The model under review builds one solid part; all positions refer to its coordinate system, in mm. A direction names the side the tool comes from. Give positions to 0.01 mm unless a question says otherwise; leave off trailing zeros. Order: outer loops, then holes, each group sorted by start corner. A loop starts at its lowest first (then second) coordinate and runs counter-clockwise, first axis right, second up. Notation, with made-up numbers: (79, 4) - (125, 4) arc R7 cw to (125, 16) - close; hole circle Ø8 at (45.25, -26). An arc over 180 degrees is marked (long way). Write item = value, one per line. Start each with the question number.
1. Machinability: for faces 1 (the cylindrical face through (8.8, -3.65, 3.67)), 2 (the flat face through (-3.8, -4.4, 0)), which of the approach directions +Z, -Z, +X, -X, +Y, -Y give a long, thin tool a straight path to every point of the face, cutting with its end or side? Answer none if there is none.
2. We need section B-B, the plane x = 0. Give the boundary of the cut face in (y, z) (3 decimals), and give its area (3 significant figures).
3. We need section C-C, the plane z = 2.7. State how many separate pieces and enclosed holes the cut face has, and give its area (3 significant figures).
4. Mouldability with a two-part tool opening along X and no side actions: class faces 3 (the flat face through (10.582, -4.532, 1.565)), 4 (the flat face through (11, 1, 3.175)), 5 (the flat face through (-15.875, 0, 2)), 6 (the cylindrical face through (-14.05, -0.06, 1.57)) as pulls with the +X half, pulls with the -X half, needs draft (parallel to the pull), parting line crosses it, or undercut.
5. For P1, Ø1.5, axis at x = 11, y = 3, coming from the +Z side (3 decimals); P2, Ø9, axis at x = 0, y = 0, coming from the -Z side, all flat-tipped, find the tip position at first contact; note any pin that passes through.
6. We need section D-D, the plane y = -4.75. Give the boundary of the cut face in (x, z) (3 decimals), and give its area (3 significant figures).
7. We need section A-A, the plane y = 0. Give the boundary of the cut face in (x, z) (3 decimals), and give its area (3 significant figures).
8. Wall thickness on probe 1 along Y at (x, z) = (12.7, 1.1) (3 decimals); probe 2 along Y at (x, z) = (0, 1.75) (3 decimals); probe 3 along Z at (x, y) = (8, 5.25) (3 decimals): over which ranges is each line inside the solid? List them lowest first.
from build123d import *

# Parameters (mm, degrees)
F0_R     = 9.525
F0_R_2   = 5.55625
F1_DEPTH = 4.445
F2_R     = 1.35255
F3_DEPTH = 3.175


with BuildPart() as f1:
    # F0 (on Top) → F1 (new body)
    with BuildSketch(Plane.XY):
        Circle(F0_R)
        Circle(F0_R_2, mode=Mode.SUBTRACT)
    extrude(amount=F1_DEPTH)

    # F2 (on face) → F3 (join)
    with BuildSketch(Plane(origin=(0, 0, 0), x_dir=(1, 0, 0), z_dir=(0, 0, -1))):
        with BuildLine():
            Line((-5.1387783316, 8.0198866737), (-12.7, 3.175))
            Line((-12.7, 3.175), (-15.875, 1.1406045195))
            Line((-15.875, 1.1406045195), (-15.875, -1.1406045195))
            Line((-15.875, -1.1406045195), (-12.7, -3.175))
            Line((-12.7, -3.175), (-5.1387783316, -8.0198866737))
            ThreePointArc((-5.1387783316, -8.0198866737), (-9.525, 0), (-5.1387783316, 8.0198866737))
        make_face()
        with Locations((-12.7, 0)):
            Circle(F2_R, mode=Mode.SUBTRACT)
        with BuildLine():
            Line((15.875, 1.1406045195), (5.1387783316, 8.0198866737))
            ThreePointArc((5.1387783316, 8.0198866737), (8.3568082606, 4.570490203), (9.525, 0))
            ThreePointArc((9.525, 0), (8.3568082606, -4.570490203), (5.1387783316, -8.0198866737))
            Line((5.1387783316, -8.0198866737), (15.875, -1.1406045195))
            Line((15.875, -1.1406045195), (15.875, 1.1406045195))
        make_face()
        with Locations((12.7, 0)):
            Circle(F2_R, mode=Mode.SUBTRACT)
    extrude(amount=-F3_DEPTH)


solid = f1.part
Model answer:
q1.face_1 = +Z
q1.face_2 = -Z, +X, -X, +Y, -Y
q2.outline = (-9.525, 0) - (-5.556, 0) - (-5.556, 4.445) - (-9.525, 4.445) - close; (5.556, 0) - (9.525, 0) - (9.525, 4.445) - (5.556, 4.445) - close
q2.area = 35.3 mm2
q3.separate_pieces = 1
q3.enclosed_holes = 3
q3.area = 274 mm2
q4.face_3 = pulls with the +X half
q4.face_4 = needs draft
q4.face_5 = pulls with the -X half
q4.face_6 = undercut
q5.P1 = 3.175
q5.P2 = through
q6.outline = (-10.242, 0) - (-2.883, 0) - (-2.883, 4.445) - (-8.256, 4.445) - (-8.256, 3.175) - (-10.242, 3.175) - close; (2.883, 0) - (10.242, 0) - (10.242, 3.175) - (8.256, 3.175) - (8.256, 4.445) - (2.883, 4.445) - close
q6.area = 60.4 mm2
q7.outline = (-15.875, 0) - (-14.053, 0) - (-14.053, 3.175) - (-15.875, 3.175) - close; (-11.347, 0) - (-5.556, 0) - (-5.556, 4.445) - (-9.525, 4.445) - (-9.525, 3.175) - (-11.347, 3.175) - close; (5.556, 0) - (11.347, 0) - (11.347, 3.175) - (9.525, 3.175) - (9.525, 4.445) - (5.556, 4.445) - close; (14.053, 0) - (15.875, 0) - (15.875, 3.175) - (14.053, 3.175) - close
q7.area = 58.4 mm2
q8.probe_1 = -3.175 to -1.353, 1.353 to 3.175
q8.probe_2 = -9.525 to -5.556, 5.556 to 9.525
q8.probe_3 = 0 to 3.175
